Verification items for the finished model (mm, model axes). A direction names the side the tool comes from. Coordinates: 2 decimals unless noted, no trailing zeros. Write each loop counter-clockwise with the first axis right and the second up, starting at its lowest first coordinate (ties: lowest second). Pieces come first, ordered by that corner, then holes. Notation, with made-up numbers: M -37,76.5 L 20,76.5 A33 ccw 20,115.5 Z; hole C -35.5,52 d10. An arc over 180 degrees is marked long. One line per item, written item: value.
Autodesk Inventor part; units mm, degrees
ref_plane "YZ Plane" through (0, 0, 0) normal (1, 0, 0) x (0, 1, 0)
ref_plane "XZ Plane" through (0, 0, 0) normal (0, 1, 0) x (-1, 0, 0)
ref_plane "XY Plane" through (0, 0, 0) normal (0, 0, 1) x (1, 0, 0)
sketch "Sketch1" plane through (0, 0, 0) normal (1, 0, 0) x (0, 1, 0)
  line L0 (0, 0) -> (0, -61)
  line L1 (0, -61) -> (20, -61)
  line L2 (20, -61) -> (20, -66)
  line L3 (20, -66) -> (-5, -66)
  line L4 (-5, -66) -> (-5, 5)
  line L5 (-5, 5) -> (20, 5)
  line L6 (20, 5) -> (20, 0)
  line L7 (20, 0) -> (0, 0)
  line L8 (0, -30.5) -> (0, -10.5)
  line L9 (0, -30.5) -> (0, -50.5)
  line L10 (0, -10.5) -> (0, -9)
  line L11 (0, -9) -> (-2.5, -9)
  line L12 (-2.5, -9) -> (-2.5, -12)
  line L13 (-2.5, -12) -> (0, -12)
  line L14 (0, -12) -> (0, -9)
  line L15 (0, -50.5) -> (0, -49)
  line L16 (0, -49) -> (-2.5, -49)
  line L17 (-2.5, -49) -> (-2.5, -52)
  line L18 (-2.5, -52) -> (0, -52)
  line L19 (0, -52) -> (0, -49)
  point P0 (0, -52)
  dimension "d0" = 61
  dimension "d1" = 20
  dimension "d2" = 5
  dimension "d3" = 25
  dimension "d4" = 71
  dimension "d7" = 20
  dimension "d8" = 20
  dimension "d9" = 1.5
  dimension "d10" = 2.5
  dimension "d11" = 3
  dimension "d12" = 1.5
  dimension "d13" = 2.5
  dimension "d14" = 3
extrude "Extrusion1" add sketch "Sketch1" along normal blind 3 contours L0 L11 L12 L13 L16 L17 L18 L1 L2 L3 L4 L5 L6 L7
properties part number "CONTAINERHOUDER LANG"
Item 1: Draft check along Z on faces 3 (the face through (1, -1, -49)), 4 (the face through (1, 20, -63)), 5 (the face through (1, 7, 5)), 6 (the face through (1, 10, 0)). Enter one of: released by +Z, released by -Z, zero draft, split by the parting line, or undercut.
The answers:
face 3: undercut
face 4: zero draft
face 5: released by +Z
face 6: undercut
Item 2: Go/stop test with flat-tipped pins: P1, Ø0.9, axis at x = 2, z = -51, coming from the +Y side; P2, Ø1, axis at x = 1.5, z = -44, coming from the +Y side. Record where each tip stops, or that it passes through.
The answers:
P1: stops at y = -2.5
P2: stops at y = 0
Item 3: Scan lines: line 1 (Z direction, x = 1.35, y = 9); line 2 (Y direction, x = 1.5, z = -9.5); line 3 (Y direction, x = 2.5, z = -53). Record each from-to range of solid material in increasing order.
The answers:
line 1: z = -66 to -61, 0 to 5
line 2: y = -5 to -2.5
line 3: y = -5 to 0
Item 4: Cross-section at C-C, the plane z = -54. Enter the section's corners in (x, y).
The answers:
outline: M 0,-5 L 3,-5 L 3,0 L 0,0 Z
Item 5: Cross-section at B-B, the plane x = 2.5. Enter the section's corners in (y, z).
The answers:
outline: M -5,-66 L 20,-66 L 20,-61 L 0,-61 L 0,-52 L -2.5,-52 L -2.5,-49 L 0,-49 L 0,-12 L -2.5,-12 L -2.5,-9 L 0,-9 L 0,0 L 20,0 L 20,5 L -5,5 Z
Item 6: Cross-section at A-A, the plane y = 10.75. Enter the section's corners in (x, z).
The answers:
outline: M 0,-66 L 3,-66 L 3,-61 L 0,-61 Z; M 0,0 L 3,0 L 3,5 L 0,5 Z
Item 7: Access from +Z, -Z, +X, -X, +Y, -Y to the whole of each face (thin tool, end or side, straight path). Record for faces 1 (the face through (3, -1, -30)), 2 (the face through (1, 10, -61)).
The answers:
face 1: +Z, -Z, +X, +Y, -Y
face 2: +X, -X, +Y
